Source: CAD feature listing. Evaluate the final solid. Frame: model axes, mm. A direction names the side the tool comes from. Round coordinates to 2 decimals unless told otherwise and drop trailing zeros. Order: outer loops, then holes, each group sorted by start corner. A loop starts at its lowest first (then second) coordinate and runs counter-clockwise, first axis right, second up. Notation, with made-up numbers: (14, 72) - (42, 72) arc R14 cw to (42, 95) - close; hole circle Ø4 at (-33.75, -13.5). An arc over 180 degrees is marked (long way). Return JSON: item names as keys, results as strings. Group by question number.
1) Ray query, line 1 (Z direction, x = -10.5, y = -6); line 2 (X direction, y = -13, z = 6.5); line 3 (Y direction, x = 10, z = 15). Return the intervals inside material, ascending. Write a range as from..to.
2) Section C-C, the plane x = -16. Return loops of the section in (y, z).
3) Contact query for flat-ended pins moving along their axis: P1, Ø4, axis at y = -25.5, z = 10, coming from the +X side; P2, Ø2, axis at y = 2.5, z = 12, coming from the +X side; P3, Ø8, axis at x = 8, z = 4, coming from the +Y side. Output: stop coordinate, or through.
4) Section B-B, the plane y = -24. Return loops of the section in (x, z), plus the area to 3 significant figures.
5) Access query for faces 1 (the cylindrical face through (6.56, -29.53, 0.75)), 2 (the flat face through (-9, -26, 20)). Directions: +Z, -Z, +X, -X, +Y, -Y. A direction counts if a zero-diameter tool reaches every point of the face in a straight line with its end or side. Return the directions, or none.
```python
from build123d import *

# Parameters (mm, degrees)
F2_ANGLE_BACK = 1.25
F2_ANGLE      = 2.5
F3_COUNT      = 8


# Not quite as in the source:
# - a feature names something its author has since deleted; it is built from what else it names


with BuildPart() as f1:
    # F0 (on Front) → F1 (revolve)
    with BuildSketch(Plane.XZ):
        Polygon((0, 0.5), (-30.25, 0.5), (-35.25, 0.5), (-35.25, 0), (0, 0), align=None)
        Polygon((-29.25, 1), (-30.25, 1), (-30.25, 0.5), (0, 0.5), (0, 1), (-27.25, 1), (-27.25, 20), (-29.25, 20), align=None)
    revolve(axis=Axis((0, 0, 0.5), (0, 0, -1)))

    # F0 (on Front) → F2 (revolve)
    with BuildSketch(Plane.XZ, mode=Mode.PRIVATE) as f2_sk:
        Polygon((-29.25, 20), (-30.25, 1), (-29.25, 1), align=None)
    revolve(f2_sk.sketch.rotate(Axis((0, 0, 0.5), (0, 0, -1)), -F2_ANGLE_BACK), axis=Axis((0, 0, 0.5), (0, 0, -1)), revolution_arc=F2_ANGLE)

    # F3: F1 ×8 about axis
    f3_axis = Axis((0, 0, 0.5), (0, 0, -1))


with BuildPart() as f1_1:
    add(f1.part)
    for i in range(1, F3_COUNT):
        add(f1.part.rotate(f3_axis, i * 360 / F3_COUNT))


solid = f1_1.part
```
Geometry check:
{
 "1": {"line 1": "0..1", "line 2": "-26.2..-23.95, 23.95..26.2", "line 3": "-27.49..-25.35, 25.35..27.49"},
 "2": {"outline": "(-31.41, 0) - (31.41, 0) - (31.41, 0.5) - (25.67, 0.5) - (25.67, 1) - (24.49, 1) - (24.49, 20) - (22.06, 20) - (22.06, 1) - (-22.06, 1) - (-22.06, 20) - (-24.49, 20) - (-24.49, 1) - (-25.67, 1) - (-25.67, 0.5) - (-31.41, 0.5) - close"},
 "3": {"P1": "x = 17.42", "P2": "x = 29.21", "P3": "y = 34.72"},
 "4": {"outline": "(-25.82, 0) - (25.82, 0) - (25.82, 0.5) - (18.41, 0.5) - (18.41, 1) - (16.72, 1) - (16.72, 20) - (12.91, 20) - (12.91, 1) - (-12.91, 1) - (-12.91, 20) - (-16.72, 20) - (-16.72, 1) - (-18.41, 1) - (-18.41, 0.5) - (-25.82, 0.5) - close", "area": "189 mm2"},
 "5": {"face 1": "+Z", "face 2": "+Z, +X, -X, +Y, -Y"}
}
